For this review, take the finished solid that the model builds, in its own axes (mm). Face numbers are marked on the shaded views. Round coordinates to 2 decimals unless told otherwise and drop trailing zeros. Loops run counter-clockwise (first coordinate to the right, second up) from the corner with the lowest first, then second, coordinate; pieces in that order, holes last. Notation, with made-up numbers: (-29.5, 87) -> (-20.5, 87) arc R17 ccw to (-20.5, 102) -> close; hole circle Ø1 at (5.25, 69.5). An arc over 180 degrees is marked (long way). Write each question's results on one line, items separated by ' | '.
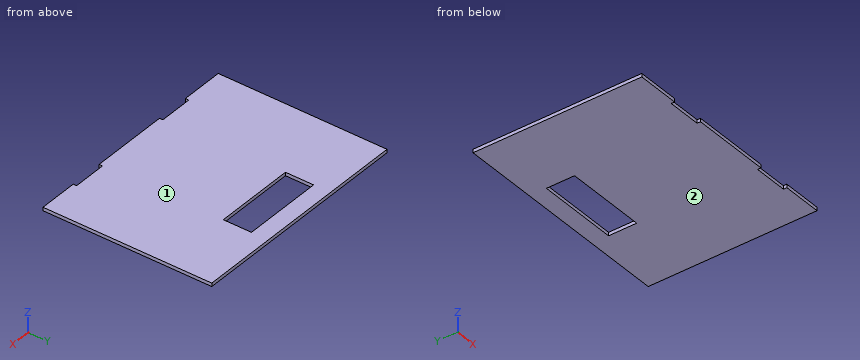
```python
from build123d import *

# Parameters (mm, degrees)
SKETCH1_W           = 203
SKETCH1_H           = 150
BOSS_EXTRUDE1_DEPTH = 3
SKETCH2_W           = 72
SKETCH2_H           = 25
CUT_EXTRUDE1_DEPTH  = 10
SKETCH3_W           = 30
SKETCH3_H           = 3
CUT_EXTRUDE2_DEPTH  = 10


with BuildPart() as part:
    # Sketch1 → Boss-Extrude1 (new body)
    with BuildSketch(Plane.XY):
        Rectangle(SKETCH1_W, SKETCH1_H)
    extrude(amount=BOSS_EXTRUDE1_DEPTH)

    # Sketch2 → Cut-Extrude1 (cut)
    with BuildSketch(Plane.XY.offset(3)):
        with Locations((0, 47.5)):
            Rectangle(SKETCH2_W, SKETCH2_H)
    extrude(amount=-CUT_EXTRUDE1_DEPTH, mode=Mode.SUBTRACT)

    # Sketch3 → Cut-Extrude2 (cut)
    with BuildSketch(Plane.XY.offset(3)):
        with Locations((-48.5, -73.5)):
            Rectangle(SKETCH3_W, SKETCH3_H)
        with Locations((51.5, -73.5)):
            Rectangle(SKETCH3_W, SKETCH3_H)
    extrude(amount=-CUT_EXTRUDE2_DEPTH, mode=Mode.SUBTRACT)


solid = part.part
```
1. To check wall thickness, follow probe 1 along X at (y, z) = (49.5, 2.3); probe 2 along Y at (x, z) = (-32, 1.1); probe 3 along Y at (x, z) = (37.5, 0.5). State the ranges of each line that lie inside material, in increasing order.
Values found:
probe 1: x = -101.5 to -36, 36 to 101.5 | probe 2: y = -75 to 35, 60 to 75 | probe 3: y = -72 to 75
2. For pin 1 (1 mm diameter, centred on x = -44, z = 1, fed in from -Y); pin 2 (1 mm diameter, centred on x = -50.5, y = 3.5, fed in from -Z), all flat-tipped, find the tip position at first contact; note any pin that passes through.
Values found:
pin 1: stops at y = -72 | pin 2: stops at z = 0
3. Consider section A-A (x = -18.5). State the section outline as (y, z) points, plus the area to 3 significant figures.
Values found:
outline: (-75, 0) -> (35, 0) -> (35, 3) -> (-75, 3) -> close; (60, 0) -> (75, 0) -> (75, 3) -> (60, 3) -> close | area: 375 mm2
4. Consider section C-C (z = 2.4). State the section outline as (x, y) points, plus the area to 3 significant figures.
Values found:
outline: (-101.5, -75) -> (-63.5, -75) -> (-63.5, -72) -> (-33.5, -72) -> (-33.5, -75) -> (36.5, -75) -> (36.5, -72) -> (66.5, -72) -> (66.5, -75) -> (101.5, -75) -> (101.5, 75) -> (-101.5, 75) -> close; hole (-36, 35) -> (36, 35) -> (36, 60) -> (-36, 60) -> close | area: 28,500 mm2
5. Consider section B-B (y = 42.5). State the section outline as (x, z) points.
Values found:
outline: (-101.5, 0) -> (-36, 0) -> (-36, 3) -> (-101.5, 3) -> close; (36, 0) -> (101.5, 0) -> (101.5, 3) -> (36, 3) -> close
6. Consider section D-D (x = -53.5). State the section outline as (y, z) points.
Values found:
outline: (-72, 0) -> (75, 0) -> (75, 3) -> (-72, 3) -> close
7. Draft analysis for pull direction Z (two halves, no side actions). For the marked faces 1 and 2, state which applies: released by +Z, released by -Z, zero draft, split by the parting line, or undercut.
Values found:
face 1: released by +Z | face 2: released by -Z
